Input: part model. Units: mm. Frame: model coordinates. A direction names the side the tool comes from. Coordinates: 2 decimals unless noted, no trailing zeros. Loops run counter-clockwise (first coordinate to the right, second up) from the corner with the lowest first, then second, coordinate; pieces in that order, holes last. Notation, with made-up numbers: (81, -23.75) - (101, -23.75) arc R7 cw to (101, -12.75) - close; hole circle Ø4 at (-29, -27). An arc over 180 degrees is marked (long way). Use a Markdown table: item, result. Add a question column.
1. Section query C-C on x = -0.75. Return the cut outline in (y, z).
2. Contact query for flat-ended pins moving along their axis: P1, Ø2, axis at x = 0, y = 0, coming from the +Z side; P2, Ø1.5, axis at x = -2.5, z = 23, coming from the +Y side; P3, Ø1.1, axis at x = 2.5, z = 22.5, coming from the -Y side. Output: stop coordinate, or through.
3. Section query B-B on z = 20. Return the cut outline in (x, y), then the cut area to 3 significant figures.
4. Draft query along Y for faces 4 (the face through (0.88, -1.56, 12.32)), 5 (the face through (3.15, 0, 8)), 6 (the face through (-1.553, 2.741, 7.745)). Return one class per face: released by +Y, released by -Y, zero draft, split by the parting line, or undercut.
5. Ray query, L1, parallel to X at y = -1, z = 1; L2, parallel to Z at x = 2.5, y = -0.75; L3, parallel to Y at x = 1.5, z = 15.5. Return the intervals inside material, ascending. Write a range as [from, to].
6. Section query A-A on y = 0.25. Return the cut outline in (x, z).
7. Access query for faces 1 (the face through (-2, -1, 23)), 2 (the face through (0, 0, -10)), 3 (the face through (0, 0, 0)). Directions: +Z, -Z, +X, -X, +Y, -Y. A direction counts if a zero-diameter tool reaches every point of the face in a straight line with its end or side. Return the directions, or none.
```python
from build123d import *

# Parameters (mm, degrees)
F1_DEPTH      = 25
F1_DEPTH_BACK = 10
F3_DEPTH      = 25
F5_DEPTH      = 13.6
F5_DEPTH_BACK = 25


with BuildPart() as f1:
    # F0 (on Top) → F1 (new body, two sides)
    with BuildSketch(Plane.XY) as f1_sk:
        Polygon((-3.15, 1.8186533479), (-3.15, -1.8186533479), (0, -3.6373066959), (3.15, -1.8186533479), (3.15, 1.8186533479), (0, 3.6373066959), align=None)
    extrude(amount=F1_DEPTH)
    extrude(f1_sk.sketch, amount=-F1_DEPTH_BACK)

    # F2 (on Top) → F3 (cut)
    with BuildSketch(Plane.XY):
        Polygon((-1.79, 1.0334569818), (-1.79, -1.0334569818), (0, -2.0669139637), (1.79, -1.0334569818), (1.79, 1.0334569818), (0, 2.0669139637), align=None)
    extrude(amount=F3_DEPTH, mode=Mode.SUBTRACT)

    # F4 (on Right) → F5 (cut, two sides)
    with BuildSketch(Plane.YZ) as f5_sk:
        Polygon((-1, 21), (0, 21), (1, 21), (1, 24), (0, 24), (-1, 24), align=None)
    extrude(amount=-F5_DEPTH, mode=Mode.SUBTRACT)
    extrude(f5_sk.sketch, amount=F5_DEPTH_BACK, mode=Mode.SUBTRACT)


solid = f1.part
```
Resolved:
| question | item | result |
|---|---|---|
| 1 | outline | (-3.2, -10) - (3.2, -10) - (3.2, 25) - (1.63, 25) - (1.63, 0) - (-1.63, 0) - (-1.63, 25) - (-3.2, 25) - close |
| 2 | P1 | z = 0 |
| 2 | P2 | y = 2.63 |
| 2 | P3 | y = -2.51 |
| 3 | outline | (-3.15, -1.82) - (0, -3.64) - (3.15, -1.82) - (3.15, 1.82) - (0, 3.64) - (-3.15, 1.82) - close; hole (-1.79, -1.03) - (0, -2.07) - (1.79, -1.03) - (1.79, 1.03) - (0, 2.07) - (-1.79, 1.03) - close |
| 3 | area | 23.3 mm² |
| 4 | face 4 | undercut |
| 4 | face 5 | zero draft |
| 4 | face 6 | released by +Y |
| 5 | L1 | [-3.15, -1.79], [1.79, 3.15] |
| 5 | L2 | [-10, 21], [24, 25] |
| 5 | L3 | [-2.77, -1.2], [1.2, 2.77] |
| 6 | outline | (-3.15, -10) - (3.15, -10) - (3.15, 21) - (1.79, 21) - (1.79, 0) - (-1.79, 0) - (-1.79, 21) - (-3.15, 21) - close; (-3.15, 24) - (-1.79, 24) - (-1.79, 25) - (-3.15, 25) - close; (1.79, 24) - (3.15, 24) - (3.15, 25) - (1.79, 25) - close |
| 7 | face 1 | +X, -X |
| 7 | face 2 | -Z, +X, -X, +Y, -Y |
| 7 | face 3 | +Z |
